Geometry check sheet. Reference: the model listing, model coordinates, mm. Round coordinates to 2 decimals unless told otherwise and drop trailing zeros. Order: outer loops, then holes, each group sorted by start corner. A loop starts at its lowest first (then second) coordinate and runs counter-clockwise, first axis right, second up.
```python
from build123d import *

# Parameters (mm, degrees)
F0_W     = 190
F0_H     = 1024
F1_DEPTH = 25
F3_DEPTH = 1024


with BuildPart() as f1:
    # F0 (on Top) → F1 (new body)
    with BuildSketch(Plane.XY):
        Rectangle(F0_W, F0_H)
    extrude(amount=F1_DEPTH)

    # F2 (on face) → F3 (cut)
    with BuildSketch(Plane.XZ.offset(512)):
        with BuildLine():
            ThreePointArc((63.386309, 25), (65.09641, 24.698463), (66.600247, 23.830222))
            Line((66.600247, 23.830222), (91.842965, 2.649067))
            ThreePointArc((91.842965, 2.649067), (92.288323, 0.98697), (90.878784, 0))
            Line((90.878784, 0), (95, 0))
            Line((95, 0), (95, 25))
            Line((95, 25), (65.20616, 25))
            Line((65.20616, 25), (63.386309, 25))
        make_face()
    extrude(amount=-F3_DEPTH, mode=Mode.SUBTRACT)


solid = f1.part
```
(1) Material ranges on line 1 (Z direction, x = 64.5, y = 344.5); line 2 (X direction, y = -464.5, z = 2.5); line 3 (X direction, y = 103.5, z = 19.5), recorded low to high.
Returned:
line 1: z = 0 to 24.87
line 2: x = -95 to 92
line 3: x = -95 to 71.76
(2) Sectioned sample at A-A, the plane y = -363. Record the cut outline in (x, z).
Returned:
outline: (-95, 0) - (90.88, 0) arc R1.5 ccw to (91.84, 2.65) - (66.6, 23.83) arc R5 ccw to (63.39, 25) - (-95, 25) - close
(3) Sectioned sample at B-B, the plane z = 20. Record the cut outline in (x, y).
Returned:
outline: (-95, -512) - (71.16, -512) - (71.16, 512) - (-95, 512) - close
